Here's how the part is built. I have some questions about the finished solid (model axes, mm). A direction names the side the tool comes from. Coordinates: 2 decimals unless noted, no trailing zeros. Use CSV: the item, a comma, the result in double quotes. Start each with the question number.
Autodesk Inventor part; units mm, degrees
ref_plane "YZ Plane" through (0, 0, 0) normal (1, 0, 0) x (0, 1, 0)
ref_plane "XZ Plane" through (0, 0, 0) normal (0, 1, 0) x (-1, 0, 0)
ref_plane "XY Plane" through (0, 0, 0) normal (0, 0, 1) x (1, 0, 0)
sketch "Sketch1" plane through (0, 0, 0) normal (0, 0, 1) x (1, 0, 0)
  line L0 (-105, -105) -> (105, -105)
  line L1 (105, -105) -> (105, 105)
  line L2 (105, 105) -> (-105, 105)
  line L3 (-105, 105) -> (-105, -105)
  line L4 (-105, -105) -> (105, 105) construction
  line L5 (105, -105) -> (-105, 105) construction
  point P0 (0, 0)
  dimension "d0" = 210
  dimension "d1" = 210
extrude "Plate1" add sketch "Sketch1" along normal mid plane 5
sketch "Sketch2" plane through (0, 0, 2.5) normal (0, 0, 1) x (1, 0, 0)
  circle A0 centre (45, 90) radius 1.65
  line L0 (105, 105) -> (105, -105)
  line L1 (105, -105) -> (-105, -105)
  line L2 (-105, 105) -> (105, 105)
  circle A1 centre (45, -92) radius 1.65
  circle A2 centre (45, -50) radius 1.65
  circle A3 centre (45, 63.5) radius 1.65
  point P0 (0, 0)
  dimension "d3" = 3.3
  dimension "d4" = 60
  dimension "d8" = 15
  dimension "d21" = 42
  dimension "d22" = 140
  dimension "d26" = 3.3
  dimension "d27" = 26.5
extrude "Cut1" cut sketch "Sketch2" against normal blind 5
sketch "Sketch3" plane through (0, 0, 2.5) normal (0, 0, 1) x (1, 0, 0)
  line L0 (-60.5, 71.35) -> (-40, 71.35)
  line L1 (-40, 71.35) -> (-40, 68.25)
  line L2 (-40, 68.25) -> (-60.5, 68.25)
  line L3 (-60.5, 68.25) -> (-60.5, 71.35)
  line L4 (0, 55.75) -> (-105, 55.75)
  line L5 (-105, 105) -> (-105, -105)
  line L6 (-50.25, 71.35) -> (-50.25, -105)
  circle A0 centre (45, 90) radius 1.65
  line L7 (105, -105) -> (-105, -105)
  line L8 (-60.5, 40.15) -> (-40, 40.15)
  line L9 (-40, 40.15) -> (-40, 43.25)
  line L10 (-40, 43.25) -> (-60.5, 43.25)
  line L11 (-60.5, 43.25) -> (-60.5, 40.15)
  point P0 (0, 0)
  point P1 (-50.25, 40.15)
  dimension "d9" = 3.1
  dimension "d11" = 20.5
  dimension "d12" = 85
  dimension "d14" = 25
  dimension "d15" = 17
extrude "Cut2" cut sketch "Sketch3" against normal blind 5 contours L0 L6 L2 L3 | L0 L1 L2 L6 | L10 L9 L8 L6 | L6 L8 L11 L10
sketch "Sketch5" plane through (0, 0, 2.5) normal (0, 0, 1) x (1, 0, 0)
  circle A0 centre (45, -50) radius 1.65
  circle A1 centre (45, -92) radius 1.65
  line L0 (45, -50) -> (45, -92)
  line L1 (39, -65) -> (51, -65)
  line L2 (51, -65) -> (51, -77)
  line L3 (51, -77) -> (39, -77)
  line L4 (39, -77) -> (39, -65)
  line L5 (39, -65) -> (51, -77) construction
  line L6 (51, -65) -> (39, -77) construction
  point P0 (0, 0)
  point P1 (45, -71)
  dimension "d23" = 12
extrude "Cut3" cut sketch "Sketch5" against normal blind 5 contours L1 L2 L3 L0 | L0 L3 L4 L1
sketch "Sketch6" plane through (0, 0, 2.5) normal (0, 0, 1) x (1, 0, 0)
  line L0 (-56.25, 61.75) -> (-44.25, 61.75)
  line L1 (-44.25, 61.75) -> (-44.25, 49.75)
  line L2 (-44.25, 49.75) -> (-56.25, 49.75)
  line L3 (-56.25, 49.75) -> (-56.25, 61.75)
  line L4 (-56.25, 61.75) -> (-44.25, 49.75) construction
  line L5 (-44.25, 61.75) -> (-56.25, 49.75) construction
  line L6 (-60.5, 71.35) -> (-40, 71.35)
  line L7 (-40, 68.25) -> (-60.5, 68.25)
  point P0 (0, 0)
  point P1 (-50.25, 55.75)
  point P2 (-50.25, 71.35)
  point P3 (-50.25, 68.25)
  dimension "d28" = 12
  dimension "d29" = 12.5
extrude "Cut4" cut sketch "Sketch6" against normal blind 5
equation "\"d6\" = Thickness"
equation "\"d17\" = Thickness"
equation "\"d24\" = Thickness"
equation "\"d30\" = Thickness"
equation "\"d2\" = Thickness"
equation "\"BendRadius\" = Thickness"
equation "\"BendReliefWidth\" = Thickness"
equation "\"BendReliefDepth\" = 0.5 * Thickness"
equation "\"TransitionRadius\" = BendRadius"
equation "\"JacobiRadiusSize\" = BendRadius"
equation "\"GapSize\" = Thickness"
properties part number "Base"
Item 1: Which directions (+Z, -Z, +X, -X, +Y, -Y) give clear straight access to the entire face, cutting with the end or side of a thin tool? Please do faces 4 (the flat face through (-50, 43.25, 0)), 5 (the flat face through (-1, 1, 2.5)).
Item 2: I'm going to push flat-ended pins straight in: pin 1 (5.5 mm diameter, centred on x = 45, y = -50, fed in from +Z); pin 2 (2 mm diameter, centred on x = 45, y = 63.5, fed in from -Z). Where does each tip first touch, or does it pass through?
Item 3: If I drill on line 1 along Y through (x, z) = (45, -1.35); line 2 along X through (y, z) = (55, 0.8); line 3 along X through (y, z) = (-66.5, -0.75), over which ranges is the centre line in solid material (lowest first)?
Item 4: Thinking about a two-plate mould opening in X: for faces 1 (the flat face through (1, 105, 0)), 2 (the flat face through (-105, 1, 0)), 3 (the flat face through (-56.25, 56, 0)), which applies, +X half, -X half, draft (parallel to the pull), parting line (faces both ways), or undercut?
Geometry says:
1,face 4,"+Z, -Z"
1,face 5,"+Z, +X, -X, +Y, -Y"
2,pin 1,"z = 2.5"
2,pin 2,"through"
3,line 1,"-105 to -93.65, -90.35 to -77, -65 to -51.65, -48.35 to 61.85, 65.15 to 88.35, 91.65 to 105"
3,line 2,"-105 to -56.25, -44.25 to 105"
3,line 3,"-105 to 39, 51 to 105"
4,face 1,"draft"
4,face 2,"-X half"
4,face 3,"undercut"
